CAD build for the part. Positions are in the model's coordinates, mm. Face numbers are marked on the shaded views. Give positions to 0.01 mm unless a question says otherwise; leave off trailing zeros. Loops run counter-clockwise (first coordinate to the right, second up) from the corner with the lowest first, then second, coordinate; pieces in that order, holes last.
Item 1: Saw through at B-B on x = 18.5. Give the cut face in (y, z), plus the area to 3 significant figures.
Item 2: Mould opens along Z. For the marked faces 1 and 2 say: released by +Z, released by -Z, zero draft, split by the parting line, or undercut.
Item 3: Probe probe 1 along Z at (x, y) = (55, 3); probe 2 along Y at (x, z) = (29, -37); probe 3 along Z at (x, y) = (46, 3.9). List the from-to ranges inside material, lowest first.
Item 4: Saw through at D-D on z = -49.5. Give the cut face in (x, y).
Item 5: Saw through at C-C on y = 1.05. Give the cut face in (x, z), plus the area to 3 significant figures.
Item 6: Saw through at A-A on z = -37.5. Give the cut face in (x, y).
Item 7: Drop flat-ended pins along their axis: P1, Ø1.5, axis at x = 35.5, z = -7, coming from the +Y side; P2, Ø1.6, axis at x = -1.5, y = 5, coming from the -Z side; P3, Ø1, axis at y = 3, z = -19, coming from the +X side. Give the stop position or say it passes through.
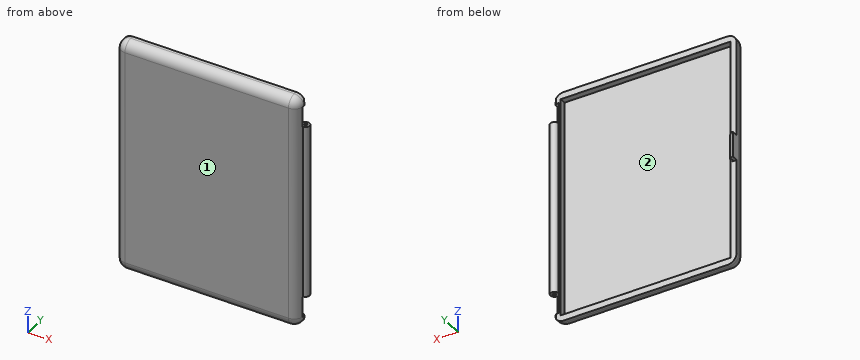
from build123d import *

# Parameters (mm, degrees)
BOTTOM_W                = 58
BOTTOM_H                = 74
BOTTOM_W_2              = 54
BOTTOM_H_2              = 70
DUVAR_DEPTH             = 4
BOTTOM_2_W              = 54
BOTTOM_2_H              = 70
TABAN_DEPTH             = 2
FILLET2_R               = 3
CENTIK_W                = 1.5
CENTIK_H                = 8
CENTIK_CIKINTI_DEPTH    = 2
SKETCH1_R               = 1.5
CUT_EXTRUDE1_DEPTH      = 6.5
CUT_EXTRUDE2_START      = -6.5
MENTESE_OUT_R           = 1.5
CUT_EXTRUDE2_DEPTH      = 6.5
BOSS_EXTRUDE3_START     = -55
SKETCH2_R               = 1.25
BOSS_EXTRUDE3_DEPTH     = 55
CUT_EXTRUDE3_DEPTH      = 92.403295892
CUT_EXTRUDE3_DEPTH_BACK = 92.403295892
MENTESE_IN_R            = 0.5
CHAMFER1_SIZE           = 1
FILLET3_R               = 1
TIRNAK_R                = 0.55
TIRNAK_EX_DEPTH         = 8


with BuildPart() as part:
    # bottom → duvar (new body)
    with BuildSketch(Plane(origin=(0, 0, 0), x_dir=(1, 0, 0), z_dir=(0, 1, 0))):
        with Locations((27, 35)):
            Rectangle(BOTTOM_W, BOTTOM_H)
        with Locations((27, 35)):
            Rectangle(BOTTOM_W_2, BOTTOM_H_2, mode=Mode.SUBTRACT)
    extrude(amount=DUVAR_DEPTH)

    # bottom<2> → taban (add)
    with BuildSketch(Plane(origin=(0, 0, 0), x_dir=(1, 0, 0), z_dir=(0, 1, 0))):
        with Locations((27, 35)):
            Rectangle(BOTTOM_2_W, BOTTOM_2_H)
    extrude(amount=TABAN_DEPTH)

    # Fillet2
    fillet2_edges = [part.edges().sort_by_distance(p)[0] for p in [
        (27, 0, -72),
        (56, 0, -35),
        (27, 0, 2),
        (-2, 0, -35),
        (-2, 2, -72),
        (56, 2, -72),
        (56, 2, 2),
        (-2, 2, 2),
    ]]
    fillet(fillet2_edges, radius=FILLET2_R)

    # centik → centik cikinti (add)
    with BuildSketch(Plane(origin=(0, 4, 0), x_dir=(1, 0, 0), z_dir=(0, 1, 0))):
        with Locations((-1.25, 35)):
            Rectangle(CENTIK_W, CENTIK_H)
    extrude(amount=CENTIK_CIKINTI_DEPTH)

    # Sketch1 → Cut-Extrude1 (cut)
    with BuildSketch(Plane.XY.offset(-1)):
        with Locations((56, 4)):
            Circle(SKETCH1_R)
    extrude(amount=-CUT_EXTRUDE1_DEPTH, mode=Mode.SUBTRACT)

    # mentese out → Cut-Extrude2 (cut)
    with BuildSketch(Plane(origin=(0, 0, -69), x_dir=(-1, 0, 0), z_dir=(0, 0, -1)).offset(CUT_EXTRUDE2_START)):
        with Locations((-56, 4)):
            Circle(MENTESE_OUT_R)
    extrude(amount=CUT_EXTRUDE2_DEPTH, mode=Mode.SUBTRACT)

    # Sketch2 → Boss-Extrude3 (add)
    with BuildSketch(Plane(origin=(0, 0, -62.5), x_dir=(-1, 0, 0), z_dir=(0, 0, -1)).offset(BOSS_EXTRUDE3_START)):
        with Locations((-56, 4)):
            Circle(SKETCH2_R)
    extrude(amount=BOSS_EXTRUDE3_DEPTH)

    # mentese in → Cut-Extrude3 (cut, two sides: drawn at the far end of the back side and taken through both)
    with BuildSketch(Plane.XY.offset(-1).offset(-CUT_EXTRUDE3_DEPTH_BACK)):
        with Locations((56, 4)):
            Circle(MENTESE_IN_R)
    extrude(amount=CUT_EXTRUDE3_DEPTH + CUT_EXTRUDE3_DEPTH_BACK, mode=Mode.SUBTRACT)

    # Chamfer1
    chamfer1_edges = [part.edges().sort_by_distance(p)[0] for p in [
        (-0.5, 6, -35),
    ]]
    chamfer(chamfer1_edges, length=CHAMFER1_SIZE)

    # Fillet3
    fillet3_edges = [part.edges().sort_by_distance(p)[0] for p in [
        (-1.5, 6, -35),
    ]]
    fillet(fillet3_edges, radius=FILLET3_R)

    # tirnak → tirnak ex (cut)
    with BuildSketch(Plane.XY.offset(-31)):
        with Locations((-0.5, 4.5)):
            Circle(TIRNAK_R)
    extrude(amount=-TIRNAK_EX_DEPTH, mode=Mode.SUBTRACT)


solid = part.part
Results below:
1. outline: (0, -69) arc R3 ccw to (3, -72) - (4, -72) - (4, -70) - (2, -70) - (2, 0) - (4, 0) - (4, 2) - (3, 2) arc R3 ccw to (0, -1) - close
1. area: 152 mm2
2. face 1: zero draft
2. face 2: undercut
3. probe 1: z = -71.24 to -69, -62.5 to -7.5, -1 to 1.24
3. probe 2: y = 0 to 2
3. probe 3: z = -72 to -70, 0 to 2
4. outline: (-2, 3) arc R3 ccw to (1, 0) - (53, 0) arc R3 ccw to (55.99, 2.75) arc R1.25 ccw (long way) to (54.75, 4) - (54, 4) - (54, 2) - (0, 2) - (0, 4) - (-2, 4) - close; hole circle Ø1 at (56, 4)
5. outline: (-1.28, -69) arc R2.28 ccw to (1, -71.28) - (53, -71.28) arc R2.28 ccw to (55.28, -69) - (55.28, -1) arc R2.28 ccw to (53, 1.28) - (1, 1.28) arc R2.28 ccw to (-1.28, -1) - close
5. area: 4,100 mm2
6. outline: (-2, 3) arc R3 ccw to (1, 0) - (53, 0) arc R3 ccw to (55.99, 2.75) arc R1.25 ccw (long way) to (54.75, 4) - (54, 4) - (54, 2) - (0, 2) - (0, 4) - (-0.27, 4) arc R0.55 cw (long way) to (-0.55, 5.05) - (-1.21, 5.71) arc R1 ccw to (-1.91, 6) - (-2, 6) - close; hole circle Ø1 at (56, 4)
7. P1: stops at y = 2
7. P2: stops at z = -39
7. P3: stops at x = 57.15
